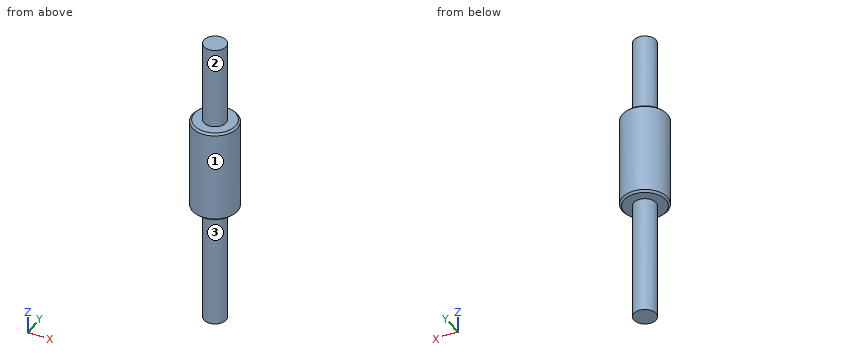
```python
from build123d import *

# Parameters (mm, degrees)
F0_R     = 2.95
F3_DEPTH = 32
F0_R_2   = 6
F4_DEPTH = 25
F2_R     = 2.95
F5_DEPTH = 22
F6_SIZE  = 0.5


with BuildPart() as f3:
    # F0 (on Top) → F3 (new body)
    with BuildSketch(Plane.XY):
        Circle(F0_R)
    extrude(amount=-F3_DEPTH)

    # F0 (on Top) → F4 (join)
    with BuildSketch(Plane.XY):
        Circle(F0_R_2)
        Circle(F0_R, mode=Mode.SUBTRACT)
        Circle(F0_R)
    extrude(amount=F4_DEPTH)

    # F2 (on offset) → F5 (join)
    with BuildSketch(Plane.XY.offset(25)):
        Circle(F2_R)
    extrude(amount=F5_DEPTH)

    # F6
    f6_edges = [f3.edges().sort_by_distance(p)[0] for p in [
        (-6, 0, 25),
        (-6, 0, 0),
    ]]
    chamfer(f6_edges, length=F6_SIZE)


solid = f3.part
```
Build history of the part. All positions in model axes, mm. Face numbers are marked on the shaded views. A direction names the side the tool comes from. Give positions to 0.01 mm unless a question says otherwise; leave off trailing zeros. Order: outer loops, then holes, each group sorted by start corner. A loop starts at its lowest first (then second) coordinate and runs counter-clockwise, first axis right, second up. Notation, with made-up numbers: M 85,45.5 L 116,45.5 A22 cw 116,51.5 Z; hole C 18.5,26.5 d10. An arc over 180 degrees is marked long. Return JSON: item names as keys, results as strings.
Q1. Band-saw the part on C-C (z = 35). Give the cut face in (x, y), then the cut area to 3 significant figures.
Answer list:
{"outline": "C 0,0 d5.9", "area": "27.3 mm^2"}
Q2. Flat gauge pins, fed straight in: pin 1 (1.5 mm diameter, centred on x = 2.5, z = 17.5, fed in from -Y); pin 2 (2 mm diameter, centred on y = -2, z = -8.5, fed in from -X); pin 3 (3 mm diameter, centred on x = -4.5, z = -5, fed in from -Y); pin 4 (5 mm diameter, centred on x = 3, z = 38, fed in from +Y). Where does each tip first touch, or does it go through?
Answer list:
{"pin 1": "stops at y = -5.74", "pin 2": "stops at x = -2.78", "pin 3": "passes through", "pin 4": "stops at y = 2.91"}
Q3. 3-axis set-ups, long thin cutter, end or side, ignore diameter. For the marked faces 1, 2 and 3: which of +Z, -Z, +X, -X, +Y, -Y reach the whole face in a straight line?
Answer list:
{"face 1": "+Z, -Z", "face 2": "+Z", "face 3": "-Z"}
Q4. Band-saw the part on A-A (y = 0). Give the cut face in (x, z), then the cut area to 3 significant figures.
Answer list:
{"outline": "M -6,0.5 L -5.5,0 L -2.95,0 L -2.95,-32 L 2.95,-32 L 2.95,0 L 5.5,0 L 6,0.5 L 6,24.5 L 5.5,25 L 2.95,25 L 2.95,47 L -2.95,47 L -2.95,25 L -5.5,25 L -6,24.5 Z", "area": "618 mm^2"}
Q5. Wall check: probe 1 along Z at (x, y) = (-1.75, -3); probe 2 along Z at (x, y) = (-3.75, 4.5); probe 3 along Y at (x, z) = (-1.25, -8). Give the ranges that are in metal, low to high. Write a range as from..to.
Answer list:
{"probe 1": "z = 0..25", "probe 2": "z = 0.36..24.64", "probe 3": "y = -2.67..2.67"}
